Can you work these out from the drawing? Everything is in mm from the part's minimum corner. A direction names the side the tool comes from. Coordinates: 2 decimals unless noted, no trailing zeros. Order: outer loops, then holes, each group sorted by start corner. A loop starts at its lowest first (then second) coordinate and runs counter-clockwise, first axis right, second up. Notation, with made-up numbers: M 19,-22 L 40,-22 A9 ccw 40,-10 Z; hole C 73.25,-31.5 d9. An arc over 180 degrees is marked long. Answer as a JSON object with one key per item and string values.
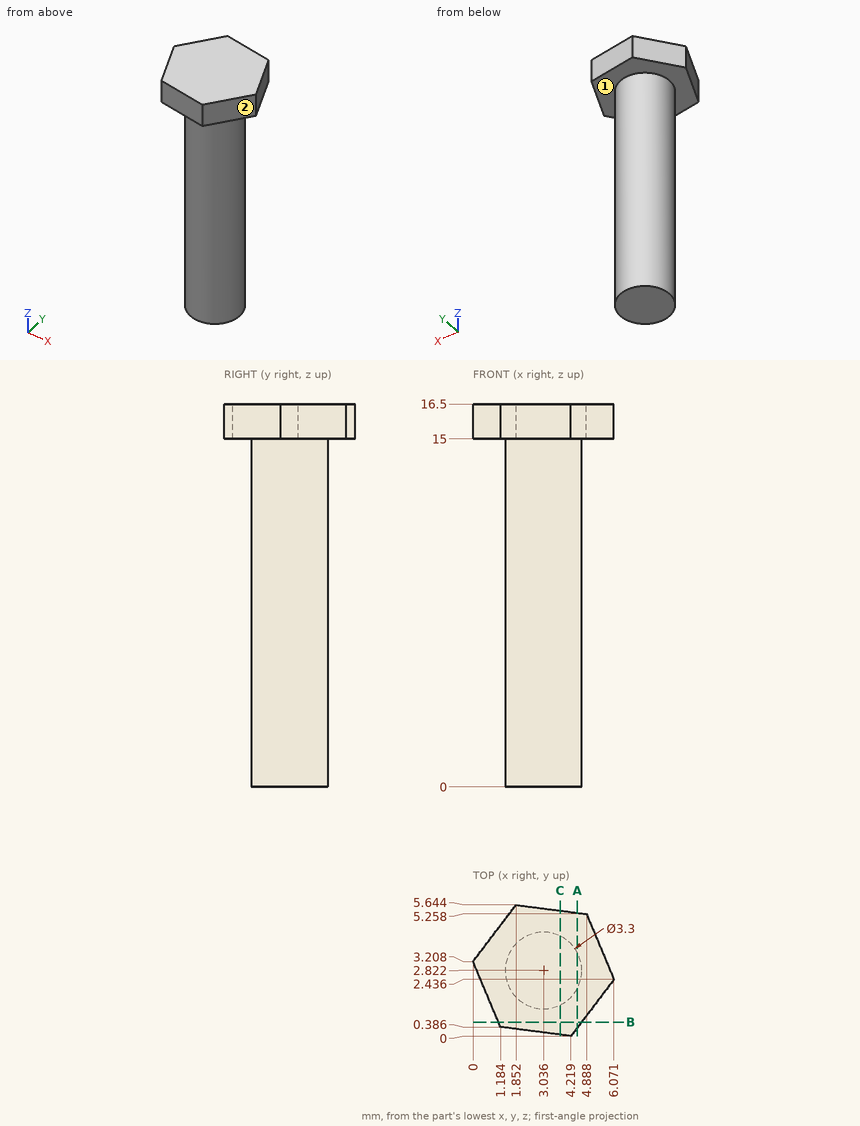
Item 1: I want a section at C-C, the plane x = 3.75. Write out the boundary of the cut face in (y, z) (1 decimal).
Answers follow:
{"outline": "M 0.1,15 L 1.3,15 L 1.3,0 L 4.3,0 L 4.3,15 L 5.4,15 L 5.4,16.5 L 0.1,16.5 Z"}
Item 2: Please list where these lines run through material, in increasing order: line 1 (X direction, y = 3, z = 14.75) (1 decimal); line 2 (Z direction, x = 3.5, y = 4.5); line 3 (X direction, y = 4.2, z = 8.5) (1 decimal).
Answers follow:
{"line 1": "x = 1.4 to 4.7", "line 2": "z = 15 to 16.5", "line 3": "x = 2.1 to 3.9"}
Item 3: I'm going to push flat-ended pins straight in: pin 1 (3 mm diameter, centred on x = 3, y = 4, fed in from -Z); pin 2 (1 mm diameter, centred on y = 1.5, z = 10.5, fed in from +X) (1 decimal); pin 3 (3 mm diameter, centred on x = 3, z = 12.5, fed in from -Y). Where does each tip first touch, or does it pass through?
Answers follow:
{"pin 1": "stops at z = 0", "pin 2": "stops at x = 4.5", "pin 3": "stops at y = 1.17"}
Item 4: I want a section at B-B, the plane y = 0.6. Write out the boundary of the cut face in (x, z) (1 decimal).
Answers follow:
{"outline": "M 1.1,15 L 4.7,15 L 4.7,16.5 L 1.1,16.5 Z"}
Item 5: I want a section at A-A, the plane x = 4.5. Write out the boundary of the cut face in (y, z).
Answers follow:
{"outline": "M 0.37,15 L 2.06,15 L 2.06,0 L 3.58,0 L 3.58,15 L 5.31,15 L 5.31,16.5 L 0.37,16.5 Z"}
Item 6: Which directions (+Z, -Z, +X, -X, +Y, -Y) give clear straight access to the entire face, cutting with the end or side of a thin tool? Please do the marked faces 1 and 2.
Answers follow:
{"face 1": "-Z", "face 2": "+Z, -Z, +X, -Y"}
